Design review of the part shown in the three views and the two pictorial views. Dimensions are in mm from the part's minimum x, y and z. Coordinates: 2 decimals unless noted, no trailing zeros. Loops run counter-clockwise (first coordinate to the right, second up) from the corner with the lowest first, then second, coordinate; pieces in that order, holes last. Notation, with made-up numbers: M 29.5,58 L 37.5,58 A25 ccw 37.5,71 Z; hole C 67,72.5 d4. An arc over 180 degrees is marked long. Answer as a JSON object with one key per item and string values. Group by question number.
Item 1: Wall thickness on L1, parallel to X at y = 0.35, z = 11; L2, parallel to X at y = 0.5, z = 0.5: over which ranges is each line inside the solid? List them lowest first. Write a range as from..to.
Item 2: Add section A-A (y = 0.55). State the section outline as (x, z) points, then the cut area to 3 significant figures.
Item 3: Add section B-B (z = 11.5). State the section outline as (x, y) points, then the cut area to 3 significant figures.
Item 4: Add section C-C (x = 19.25). State the section outline as (y, z) points, then the cut area to 3 significant figures.
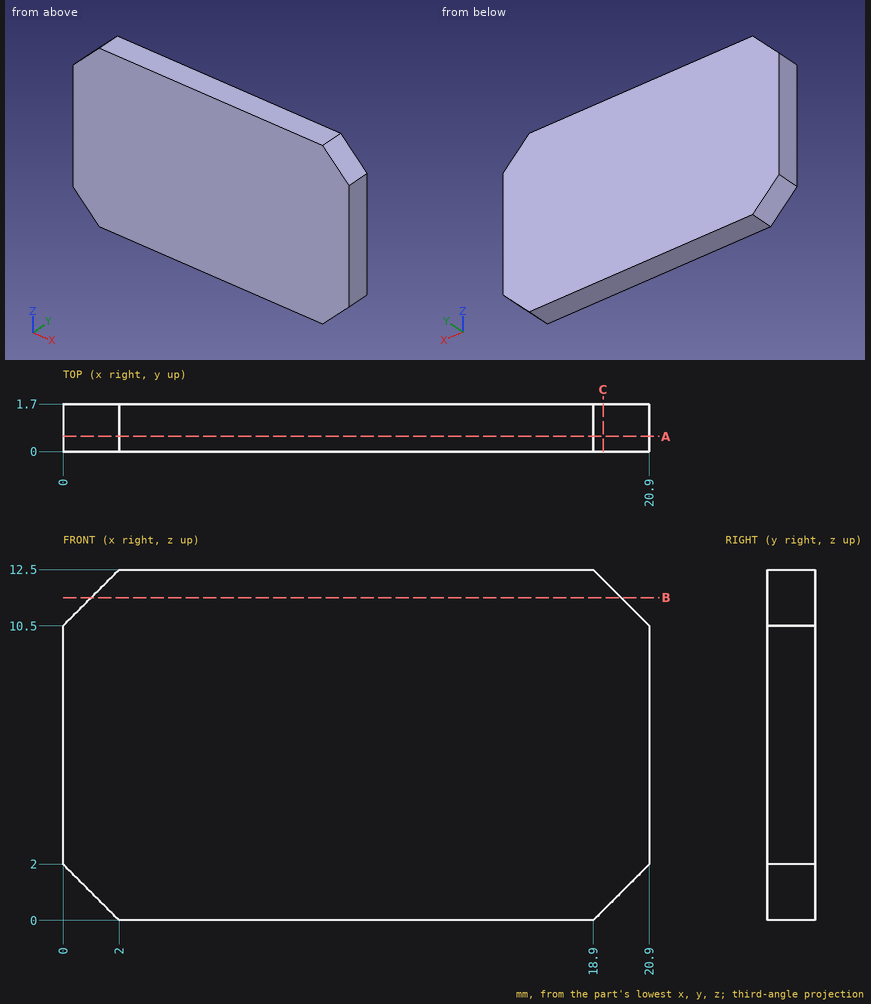
From the geometry:
{
 "1": {"L1": "x = 0.5..20.4", "L2": "x = 1.5..19.4"},
 "2": {"outline": "M 0,2 L 2,0 L 18.9,0 L 20.9,2 L 20.9,10.5 L 18.9,12.5 L 2,12.5 L 0,10.5 Z", "area": "253 mm²"},
 "3": {"outline": "M 1,0 L 19.9,0 L 19.9,1.7 L 1,1.7 Z", "area": "32.1 mm²"},
 "4": {"outline": "M 0,0.35 L 1.7,0.35 L 1.7,12.15 L 0,12.15 Z", "area": "20.1 mm²"}
}
